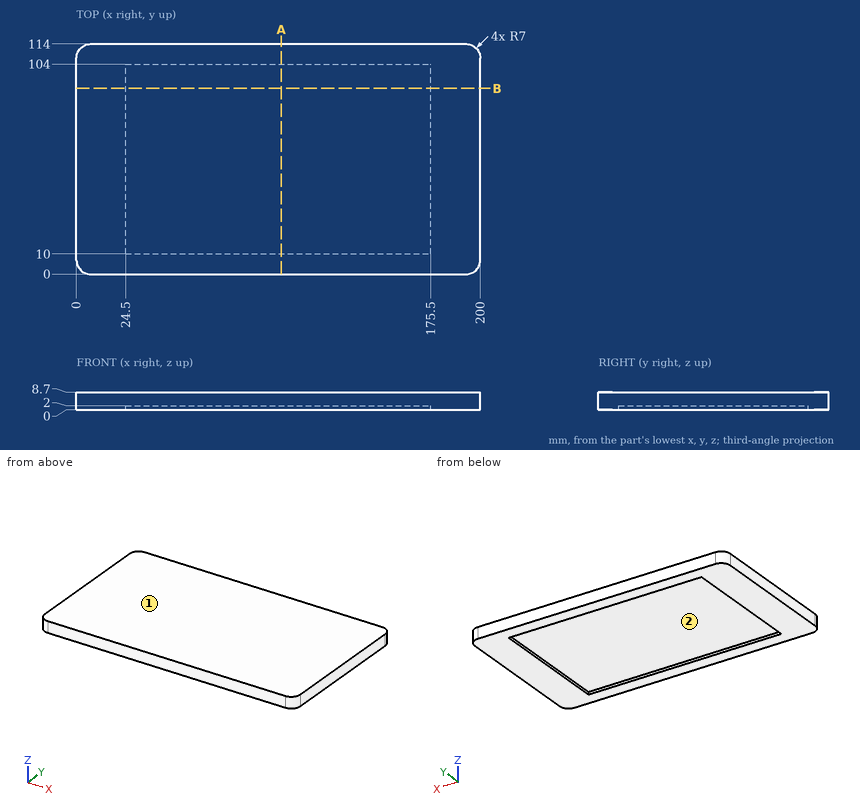
Design review of the part shown in the three views and the two pictorial views. Dimensions are in mm from the part's minimum x, y and z. Give positions to 0.01 mm unless a question says otherwise; leave off trailing zeros. Loops run counter-clockwise (first coordinate to the right, second up) from the corner with the lowest first, then second, coordinate; pieces in that order, holes last. Notation, with made-up numbers: M 43,-35.75 L 88,-35.75 A15 ccw 88,-16.75 Z; hole C 57.5,72.5 d11. An arc over 180 degrees is marked long. Put each result on its own line as item: value. Start each with the question number.
(1) For pin 1 (12 mm diameter, centred on x = 166.5, y = 85, fed in from -Z), flat-tipped, find the tip position at first contact; note if it passes through.
(2) Add section A-A, the plane x = 101.5. Write out the cut boundary in (y, z), then the cut area to 3 significant figures.
(3) The part is to be moulded in two halves that separate along X. For the marked faces 1 and 2, say which applies: +X half, -X half, draft (parallel to the pull), parting line (faces both ways), or undercut.
(4) Wall thickness on L1, parallel to X at y = 64.5, z = 0.5; L2, parallel to Y at x = 123, z = 1.5; L3, parallel to Z at x = 166, y = 49.5: over which ranges is each line inside the solid? List them lowest first.
(5) Add section B-B, the plane y = 92. Write out the cut boundary in (x, z).
Result:
1. pin 1: stops at z = 2
2. outline: M 0,0 L 10,0 L 10,2 L 104,2 L 104,0 L 114,0 L 114,8.7 L 0,8.7 Z
2. area: 804 mm^2
3. face 1: draft
3. face 2: undercut
4. L1: x = 0 to 24.5, 175.5 to 200
4. L2: y = 0 to 10, 104 to 114
4. L3: z = 2 to 8.7
5. outline: M 0,0 L 24.5,0 L 24.5,2 L 175.5,2 L 175.5,0 L 200,0 L 200,8.7 L 0,8.7 Z
